Build history of the part. All positions in model axes, mm. Face numbers are marked on the shaded views. A direction names the side the tool comes from. Coordinates: 2 decimals unless noted, no trailing zeros. Order: outer loops, then holes, each group sorted by start corner. A loop starts at its lowest first (then second) coordinate and runs counter-clockwise, first axis right, second up. Notation, with made-up numbers: (-10, 18.25) - (14, 18.25) arc R24 ccw to (14, 50.25) - close; hole circle Ø10 at (75, -5.75). An arc over 180 degrees is marked (long way). Write each question's results on one line, items separated by ' | '. Start each with the question number.
from build123d import *

# Parameters (mm, degrees)
F1_DEPTH = 25.4


with BuildPart() as f1:
    # F0 (on Front) → F1 (new body)
    with BuildSketch(Plane.XZ):
        Polygon((35.668362, 43.594655), (-36.028642, 43.594655), (-36.028642, 19.095179), (-21.538323, 19.095179), (21.042599, 19.095179), (35.668362, 19.095179), align=None)
        with BuildLine():
            Line((-21.538323, 19.095179), (-36.028642, 19.095179))
            Line((-36.028642, 19.095179), (-23.710124, -8.205322))
            ThreePointArc((-23.710124, -8.205322), (-22.304387, -9.838812), (-20.237289, -10.448311))
            Line((-20.237289, -10.448311), (19.210294, -10.448311))
            ThreePointArc((19.210294, -10.448311), (21.245158, -9.859402), (22.650968, -8.274729))
            Line((22.650968, -8.274729), (35.668362, 19.095179))
            Line((35.668362, 19.095179), (21.042599, 19.095179))
            Line((21.042599, 19.095179), (13.273281, 2.759688))
            Line((13.273281, 2.759688), (-14.16743, 2.759688))
            Line((-14.16743, 2.759688), (-21.538323, 19.095179))
        make_face()
    extrude(amount=F1_DEPTH)


solid = f1.part
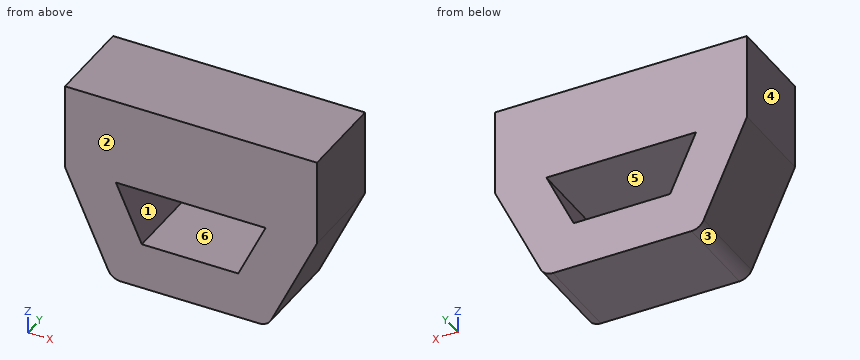
Item 1: Pull direction Z, two halves, no side cores. Call the marked faces 3, 4, 5 and 6: released by +Z, released by -Z, zero draft, split by the parting line, or undercut.
Item 2: Slice it at C-C (z = 12.5). Write the cut outline in (x, y), then the cut area to 3 significant figures.
Item 3: Probe probe 1 along Z at (x, y) = (-5.5, -18.75); probe 2 along Z at (x, y) = (17.5, -5.5); probe 3 along X at (y, z) = (-15.75, 13). List the from-to ranges inside material, lowest first.
Item 4: Slice it at A-A (x = 8). Write the cut outline in (y, z), then the cut area to 3 significant figures.
Item 5: Flat gauge pin, fed straight in: P1, Ø6, axis at y = -5.5, z = -0.5, coming from the -X side. Where does the tip first touch, or does it go through?
Item 6: Slice it at B-B (y = -6). Write the cut outline in (x, z), then the cut area to 3 significant figures.
Item 7: Slice it at D-D (z = -6). Write the cut outline in (x, y), then the cut area to 3 significant figures.
Item 8: Which spindle directions (+Z, -Z, +X, -X, +Y, -Y) get a long thin tool onto all of the face, cutting with end or side? Do the marked faces 1 and 2. Say none if no direction does.
Resolved:
1) face 3: released by -Z | face 4: zero draft | face 5: undercut | face 6: undercut
2) outline: (-33.05, -25.4) - (-18.56, -25.4) - (-18.56, 0) - (-33.05, 0) - close; (17.91, -25.4) - (32.53, -25.4) - (32.53, 0) - (17.91, 0) - close | area: 740 mm^2
3) probe 1: -10.45 to 2.76, 19.1 to 43.59 | probe 2: -10.45 to 11.65, 19.1 to 43.59 | probe 3: -33.28 to -18.79, 18.14 to 32.77
4) outline: (-25.4, -10.45) - (0, -10.45) - (0, 2.76) - (-25.4, 2.76) - close; (-25.4, 19.1) - (0, 19.1) - (0, 43.59) - (-25.4, 43.59) - close | area: 958 mm^2
5) P1: x = -28.54
6) outline: (-36.03, 19.1) - (-23.71, -8.21) arc R3.81 ccw to (-20.24, -10.45) - (19.21, -10.45) arc R3.81 ccw to (22.65, -8.27) - (35.67, 19.1) - (35.67, 43.59) - (-36.03, 43.59) - close; hole (-21.54, 19.1) - (-14.17, 2.76) - (13.27, 2.76) - (21.04, 19.1) - close | area: 2,900 mm^2
7) outline: (-24.71, -25.4) - (23.73, -25.4) - (23.73, 0) - (-24.71, 0) - close | area: 1,230 mm^2
8) face 1: +Y, -Y | face 2: +Z, -Z, +X, -X, -Y
